Drawing for the job (mm, zero at the part's lowest x, y, z). A direction names the side the tool comes from. Round coordinates to 2 decimals unless told otherwise and drop trailing zeros. Write each loop counter-clockwise with the first axis right and the second up, starting at its lowest first coordinate (ties: lowest second). Pieces come first, ordered by that corner, then holes. Notation, with made-up numbers: (54, 52) -> (82, 52) arc R13 cw to (82, 72) -> close; hole circle Ø11 at (58, 39.25). An arc over 180 degrees is marked (long way). One line per question, with ' | ' between items.
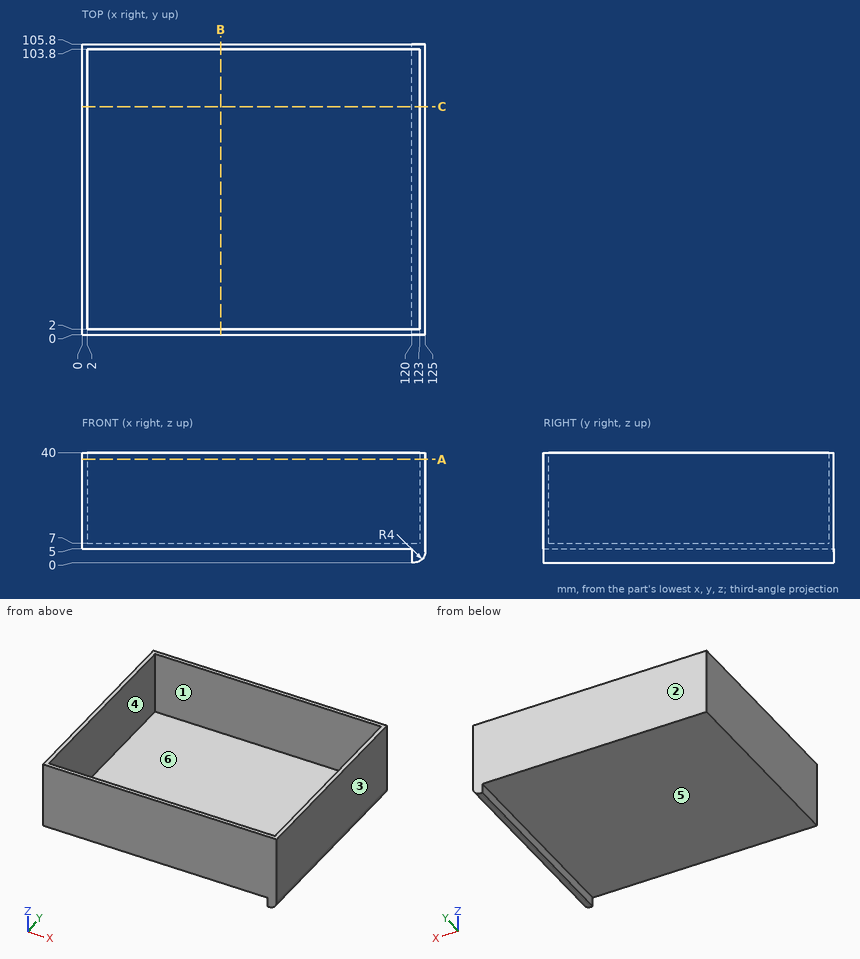
(1) Slice it at A-A (z = 37.5). Write the cut outline in (x, y), then the cut area to 3 significant figures.
Calculated:
outline: (0, 0) -> (125, 0) -> (125, 105.8) -> (0, 105.8) -> close; hole (2, 2) -> (123, 2) -> (123, 103.8) -> (2, 103.8) -> close | area: 907 mm2
(2) Slice it at C-C (y = 83). Write the cut outline in (x, z).
Calculated:
outline: (0, 5) -> (120, 5) -> (120, 0) -> (121, 0) arc R4 ccw to (125, 4) -> (125, 40) -> (123, 40) -> (123, 7) -> (2, 7) -> (2, 40) -> (0, 40) -> close
(3) Wall check: line 1 (X direction, y = 34.5, z = 21.5); line 2 (Y direction, x = 91.5, z = 19); line 3 (Z direction, x = 27.5, y = 87.5). Give the ranges that are in metal, low to high. Write a range as from..to.
Calculated:
line 1: 0..2, 123..125 | line 2: 0..2, 103.8..105.8 | line 3: 5..7
(4) 3-axis set-ups, long thin cutter, end or side, ignore diameter. For the marked faces 1 and 2: which of +Z, -Z, +X, -X, +Y, -Y reach the whole face in a straight line?
Calculated:
face 1: +Z | face 2: +Z, -Z, +X, -X, +Y
(5) Drop flat-ended pins along their axis: pin 1 (12 mm diameter, centred on x = 93.5, z = 22.5, fed in from -Y); pin 2 (1 mm diameter, centred on x = 82, y = 66.5, fed in from -Z); pin 3 (1.5 mm diameter, centred on x = 71, y = 18, fed in from +Z). Give the stop position or say it passes through.
Calculated:
pin 1: y = 0 | pin 2: z = 5 | pin 3: z = 7
(6) Slice it at B-B (x = 50.5). Write the cut outline in (y, z).
Calculated:
outline: (0, 5) -> (105.8, 5) -> (105.8, 40) -> (103.8, 40) -> (103.8, 7) -> (2, 7) -> (2, 40) -> (0, 40) -> close
(7) Mould opens along X. For the marked faces 3, 4, 5 and 6 say: pulls with the +X half, pulls with the -X half, needs draft (parallel to the pull), parting line crosses it, or undercut.
Calculated:
face 3: pulls with the +X half | face 4: undercut | face 5: needs draft | face 6: undercut
